Geometry: final body of the model. Coordinates: model frame, mm. Round coordinates to 2 decimals unless told otherwise and drop trailing zeros. Write each loop counter-clockwise with the first axis right and the second up, starting at its lowest first coordinate (ties: lowest second). Pieces come first, ordered by that corner, then holes.
Autodesk Inventor part; units mm, degrees
ref_plane "YZ Plane" through (0, 0, 0) normal (1, 0, 0) x (0, 1, 0)
ref_plane "XZ Plane" through (0, 0, 0) normal (0, 1, 0) x (-1, 0, 0)
ref_plane "XY Plane" through (0, 0, 0) normal (0, 0, 1) x (1, 0, 0)
sketch "Sketch1" plane through (0, 0, 0) normal (0, 0, 1) x (1, 0, 0)
  line L0 (-31.75, 31.75) -> (31.75, 31.75)
  line L1 (31.75, 31.75) -> (31.75, -31.75)
  line L2 (31.75, -31.75) -> (-31.75, -31.75)
  line L3 (-31.75, -31.75) -> (-31.75, 31.75)
  line L4 (0, 0) -> (31.75, 0) construction
  line L5 (0, 0) -> (-31.75, 0) construction
  line L6 (0, 0) -> (0, 31.75) construction
  line L7 (0, 0) -> (0, -31.75) construction
  dimension "d0" = 63.5
  dimension "d1" = 63.5
extrude "Extrusion1" add sketch "Sketch1" along normal mid plane 3.7
sketch "Sketch2" plane through (0, 0, 1.85) normal (0, 0, 1) x (1, 0, 0)
  point P0 (0, 0)
hole "Hole1" at (0, 0, 1.85) direction (0, 0, -1) diameter 40.45 end through all
sketch "Sketch3" plane through (0, 0, 1.85) normal (0, 0, 1) x (1, 0, 0)
  circle A0 centre (0, 0) radius 20.225
  point P0 (0, 25.4)
  dimension "d11" = 25.4
hole "Hole2" at (0, 25.4, 1.85) direction (0, 0, -1) diameter 5 end through all
pattern_circular "Circular Pattern1" count 4 over 360 about axis through (0, 0, -88.0288) along (0, 0, 1) of "Hole2"
sketch "Sketch4" plane through (0, 0, 1.85) normal (0, 0, 1) x (1, 0, 0)
  circle A0 centre (-25.4, 0) radius 2.5
  circle A1 centre (0, 25.4) radius 2.5
  point P0 (-25, 24.8272)
  dimension "d24" = 24.8272
  dimension "d25" = 25
hole "Hole3" at (-25, 24.8272, 1.85) direction (0, 0, -1) diameter 2.459 end through all
pattern_circular "Circular Pattern2" count 4 over 360 about axis through (0, 0, -88.0288) along (0, 0, 1) of "Hole3"
fillet "Fillet1" radius 1 4 edges at (-31.75, 31.75, 0) (-31.75, -31.75, 0) (31.75, -31.75, 0) (31.75, 31.75, 0)
properties part number "BB2-InterfacePlate" material "Aluminum-6061"
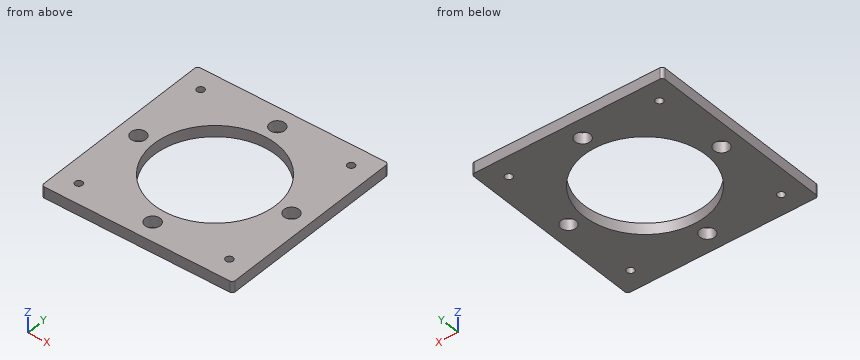
1) Section A-A on y = 0. Output: boundary loops of the cut face in (x, z) (3 decimals), plus the area to 3 significant figures.
2) Line query: probe 1 along Y at (x, z) = (-1, -0.65); probe 2 along X at (y, z) = (25.4, -0.85); probe 3 along Y at (x, z) = (-25, 0.9). Output: solid intervals per line, ascending.
3) Section D-D on y = 13. Output: boundary loops of the cut face in (x, z).
4) Section C-C on x = -16. Output: boundary loops of the cut face in (y, z).
5) Section B-B on z = -0.7. State how many separate pieces and enclosed holes the cut face has, plus the area to 3 significant figures.
Filled in:
1. outline: (-31.75, -1.85) - (-27.9, -1.85) - (-27.9, 1.85) - (-31.75, 1.85) - close; (-22.9, -1.85) - (-20.225, -1.85) - (-20.225, 1.85) - (-22.9, 1.85) - close; (20.225, -1.85) - (22.9, -1.85) - (22.9, 1.85) - (20.225, 1.85) - close; (27.9, -1.85) - (31.75, -1.85) - (31.75, 1.85) - (27.9, 1.85) - close
1. area: 48.3 mm2
2. probe 1: y = -31.75 to -27.69, -23.11 to -20.2, 20.2 to 23.11, 27.69 to 31.75
2. probe 2: x = -31.75 to -26.09, -23.91 to -2.5, 2.5 to 23.66, 25.99 to 31.75
2. probe 3: y = -31.75 to -26.22, -23.78 to -2.47, 2.47 to 23.6, 26.06 to 31.75
3. outline: (-31.75, -1.85) - (-15.49, -1.85) - (-15.49, 1.85) - (-31.75, 1.85) - close; (15.49, -1.85) - (31.75, -1.85) - (31.75, 1.85) - (15.49, 1.85) - close
4. outline: (-31.75, -1.85) - (-12.37, -1.85) - (-12.37, 1.85) - (-31.75, 1.85) - close; (12.37, -1.85) - (31.75, -1.85) - (31.75, 1.85) - (12.37, 1.85) - close
5. separate pieces: 1
5. enclosed holes: 9
5. area: 2,650 mm2
